Autodesk Inventor part; units mm, degrees
ref_plane "YZ Plane" through (0, 0, 0) normal (1, 0, 0) x (0, 1, 0)
ref_plane "XZ Plane" through (0, 0, 0) normal (0, 1, 0) x (-1, 0, 0)
ref_plane "XY Plane" through (0, 0, 0) normal (0, 0, 1) x (1, 0, 0)
sketch "Sketch1" plane through (0, 0, 0) normal (0, 0, 1) x (1, 0, 0)
  line L0 (11.825, -16.125) -> (-11.825, -16.125)
  line L1 (-14.625, -13.325) -> (-14.625, 16.125)
  line L2 (-14.625, 16.125) -> (14.625, 16.125)
  line L3 (14.625, 16.125) -> (14.625, -13.325)
  line L4 (14.625, -16.125) -> (-14.625, 16.125) construction
  line L5 (-14.625, -16.125) -> (14.625, 16.125) construction
  line L6 (11.825, -16.125) -> (14.625, -13.325)
  line L7 (-14.625, -13.325) -> (-14.625, -16.125)
  line L8 (-14.625, -16.125) -> (-11.825, -16.125)
  point P0 (0, 0)
  dimension "d0" = 29.25
  dimension "d1" = 32.25
  dimension "d24" = 2.8
  dimension "d25" = 2.8
extrude "Extrusion1" add sketch "Sketch1" along normal blind 5
shell "Shell2" thickness 5 outward yes removed faces 1 at (-4.875, -3.5083, 5)
sketch "Sketch3" plane through (0, 0, 5) normal (0, 0, 1) x (1, 0, 0)
  line L0 (19.625, 21.125) -> (-19.625, 21.125) construction
  line L1 (-14.625, 16.125) -> (14.625, 16.125) construction
  line L2 (-19.625, 21.125) -> (-14.625, 16.125) construction
  line L3 (19.625, -15.3961) -> (19.625, 21.125) construction
  line L4 (14.625, 16.125) -> (19.625, 21.125) construction
  line L5 (11.825, -16.125) -> (-14.625, -16.125) construction
  circle A0 centre (-17.125, 18.625) radius 1.25
  circle A1 centre (17.125, 18.625) radius 1.25
  line L6 (-14.625, -16.125) -> (11.825, -16.125) construction
  line L7 (-19.625, 21.125) -> (-19.625, -21.125) construction
  line L8 (-14.625, -16.125) -> (-19.625, -21.125) construction
  circle A2 centre (-17.125, -18.625) radius 1.25
  point P0 (0, 0)
  point P1 (-11.825, -16.125)
  dimension "d14" = 2.5
  dimension "d15" = 2.5
  dimension "d26" = 2.5
extrude "Extrusion3" cut sketch "Sketch3" against normal through all
sketch "Sketch4" plane through (0, 0, 5) normal (0, 0, 1) x (1, 0, 0)
  line L0 (-19.625, -21.125) -> (13.8961, -21.125)
  line L1 (11.825, -16.125) -> (-14.625, -16.125)
  line L2 (7.625, -21.125) -> (-12.375, -21.125)
  line L3 (-12.375, -21.125) -> (-12.375, -16.125)
  line L4 (-12.375, -16.125) -> (7.625, -16.125)
  line L5 (7.625, -16.125) -> (7.625, -21.125)
  line L6 (-19.625, 21.125) -> (-19.625, -21.125)
  point P0 (0, 0)
  point P1 (-13.4819, -20.125)
  point P2 (14.625, -16.125)
  point P3 (-11.825, -16.125)
  point P4 (7.625, -16.125)
  point P5 (13.8961, -21.125)
  dimension "d19" = 20
  dimension "d20" = 5
  dimension "d29" = 7.25
extrude "Extrusion4" cut sketch "Sketch4" against normal blind 4
sketch "Sketch5" plane through (0, 0, -5) normal (0, 0, -1) x (-1, 0, 0)
  line L0 (-19.625, 21.125) -> (19.625, 21.125)
  line L1 (19.625, -21.125) -> (-13.8961, -21.125)
  line L2 (-19.625, 21.125) -> (19.625, 21.125)
  line L3 (19.625, 21.125) -> (19.625, -21.125)
  line L4 (19.625, -21.125) -> (-19.625, -21.125)
  line L5 (-19.625, -21.125) -> (-19.625, 21.125)
  point P0 (0, 0)
  point P1 (19.625, 21.125)
extrude "Extrusion5" cut sketch "Sketch5" against normal blind 2
equation "\"d25\" = d24"
equation "\"d26\" = d14"
properties part number "SpeakerHolder"
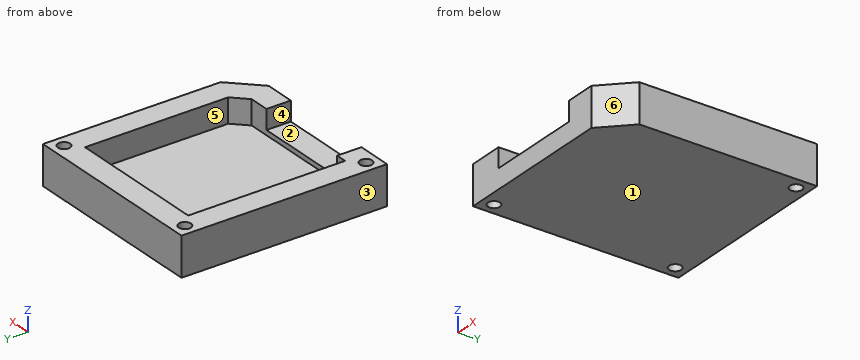
For this review, take the finished solid that the model builds, in its own axes (mm). Face numbers are marked on the shaded views. A direction names the side the tool comes from. Round coordinates to 2 decimals unless told otherwise and drop trailing zeros. Loops run counter-clockwise (first coordinate to the right, second up) from the corner with the lowest first, then second, coordinate; pieces in that order, holes last. Notation, with made-up numbers: (55, -14.5) - (95, -14.5) arc R27 cw to (95, 10.5) - close; hole circle Ø4 at (64.25, 27.5). An arc over 180 degrees is marked (long way). Use one line per item in the form item = value.
1) Tool access review of the marked faces 4, 5 and 6: name each direction out of +Z, -Z, +X, -X, +Y, -Y from which nothing blocks a thin tool from reaching the whole face with its end or side.
Solutions:
face_4 = +Z, -Y
face_5 = +Z
face_6 = +Z, -Z, +X, -Y
2) We need section D-D on z = -2. Write out the cut boundary in (x, y) (3 decimals), then the cut area to 3 significant figures.
Solutions:
outline = (-19.625, -21.125) - (13.896, -21.125) - (19.625, -15.396) - (19.625, 21.125) - (-19.625, 21.125) - close; hole circle Ø2.5 at (-17.125, -18.625); hole circle Ø2.5 at (-17.125, 18.625); hole circle Ø2.5 at (17.125, 18.625)
area = 1,630 mm2
3) Wall thickness on probe 1 along X at (y, z) = (18.5, -1) (3 decimals); probe 2 along X at (y, z) = (-12, 4) (3 decimals); probe 3 along Y at (x, z) = (-14, 3.25) (3 decimals): over which ranges is each line inside the solid? List them lowest first.
Solutions:
probe_1 = -19.625 to -18.369, -15.881 to 15.881, 18.369 to 19.625
probe_2 = -19.625 to -14.625, 14.625 to 19.625
probe_3 = -21.125 to -16.125, 16.125 to 21.125
4) We need section B-B on z = 2.5. Write out the cut boundary in (x, y) (3 decimals).
Solutions:
outline = (-19.625, -21.125) - (-12.375, -21.125) - (-12.375, -16.125) - (-14.625, -16.125) - (-14.625, 16.125) - (14.625, 16.125) - (14.625, -13.325) - (11.825, -16.125) - (7.625, -16.125) - (7.625, -21.125) - (13.896, -21.125) - (19.625, -15.396) - (19.625, 21.125) - (-19.625, 21.125) - close; hole circle Ø2.5 at (-17.125, -18.625); hole circle Ø2.5 at (-17.125, 18.625); hole circle Ø2.5 at (17.125, 18.625)
5) We need section C-C on y = -9.5. Write out the cut boundary in (x, z) (3 decimals), then the cut area to 3 significant figures.
Solutions:
outline = (-19.625, -3) - (19.625, -3) - (19.625, 5) - (14.625, 5) - (14.625, 0) - (-14.625, 0) - (-14.625, 5) - (-19.625, 5) - close
area = 168 mm2
6) Clearance check with flat-ended pins moving along their axes: P1, Ø2, axis at x = 17.125, y = 18.625, coming from the -Z side; P2, Ø2, axis at x = 10.5, y = -0.5, coming from the +Z side; P3, Ø3, axis at y = -18.5, z = 2, coming from the +X side; P4, Ø2.5, axis at x = 0, y = -19.5, coming from the +Z side. State where each tip first meets the part, or that it passes through.
Solutions:
P1 = through
P2 = 0
P3 = 18.02
P4 = 1
7) We need section A-A on x = 5. Write out the cut boundary in (y, z) (3 decimals).
Solutions:
outline = (-21.125, -3) - (21.125, -3) - (21.125, 5) - (16.125, 5) - (16.125, 0) - (-16.125, 0) - (-16.125, 1) - (-21.125, 1) - close
8) Mouldability with a two-part tool opening along X and no side actions: class the marked faces 1, 2 and 3 as pulls with the +X half, pulls with the -X half, needs draft (parallel to the pull), parting line crosses it, or undercut.
Solutions:
face_1 = needs draft
face_2 = undercut
face_3 = pulls with the -X half
